Autodesk Inventor part; units mm, degrees
ref_plane "YZ Plane" through (0, 0, 0) normal (1, 0, 0) x (0, 1, 0)
ref_plane "XZ Plane" through (0, 0, 0) normal (0, 1, 0) x (-1, 0, 0)
ref_plane "XY Plane" through (0, 0, 0) normal (0, 0, 1) x (1, 0, 0)
sketch "Sketch1" plane through (0, 0, 0) normal (0, 1, 0) x (-1, 0, 0)
  line L0 (-25.4, -7.9375) -> (25.4, -7.9375)
  line L1 (25.4, -7.9375) -> (25.4, 7.9375)
  line L2 (25.4, 7.9375) -> (-25.4, 7.9375)
  line L3 (-25.4, 7.9375) -> (-25.4, -7.9375)
  line L4 (-25.4, -7.9375) -> (25.4, 7.9375) construction
  line L5 (25.4, -7.9375) -> (-25.4, 7.9375) construction
  point P0 (0, 0)
  dimension "d0" = 50.8
  dimension "d1" = 15.875
extrude "Extrusion1" add sketch "Sketch1" along normal blind 9.525
sketch "Sketch2" plane through (-25.4, 0, -7.9375) normal (-1, 0, 0) x (0, 0, 1)
  line L0 (0, 9.525) -> (15.875, 9.525)
  line L1 (9.5418, 3.175) -> (6.3668, 3.175)
  line L2 (6.3668, 3.175) -> (6.3668, 9.525)
  line L3 (6.3668, 9.525) -> (9.5418, 9.525)
  line L4 (9.5418, 9.525) -> (9.5418, 3.175)
  line L5 (9.5418, 3.175) -> (6.3668, 9.525) construction
  line L6 (6.3668, 3.175) -> (9.5418, 9.525) construction
  point P0 (7.9375, 0)
  point P1 (7.9543, 6.35)
  dimension "d4" = 3.175
  dimension "d5" = 6.35
extrude "Extrusion2" cut sketch "Sketch2" against normal up to next
properties part number "Test1"
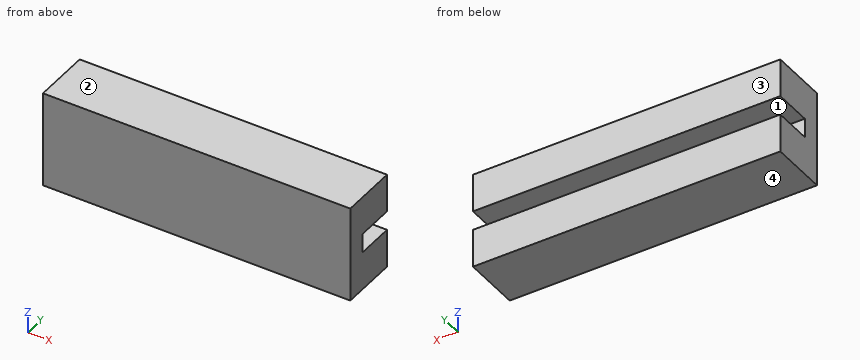
The model under review builds one solid part; all positions refer to its coordinate system, in mm. Face numbers are marked on the shaded views. Round coordinates to 2 decimals unless told otherwise and drop trailing zeros. Order: outer loops, then holes, each group sorted by start corner. A loop starts at its lowest first (then second) coordinate and runs counter-clockwise, first axis right, second up. Notation, with made-up numbers: (86.25, 26.25) -> (127.25, 26.25) arc R24 ccw to (127.25, 62.25) -> close; hole circle Ø9 at (0, -35). An arc over 180 degrees is marked (long way). One line per item, written item: value. Start each with the question number.
Q1. Wall thickness on line 1 (Z direction, x = 16, y = 8.75); line 2 (Y direction, x = -3, z = 1.5) (3 decimals): over which ranges is each line inside the solid? List them lowest first.
Q2. Clearance check with flat-ended pins moving along their axes: pin 1 Ø1.6 at (x, z) = (-9, -0.5) entering from +Y (3 decimals); pin 2 Ø8 at (x, z) = (3.5, -4.5) entering from -Y. State where each tip first meets the part, or that it passes through.
Q3. Take a section at C-C (z = -0.75). Write out the cut boundary in (x, y) (3 decimals).
Q4. Take a section at A-A (y = 8.5). Write out the cut boundary in (x, z), and give its area (3 significant figures).
Q5. Mouldability with a two-part tool opening along Z and no side actions: class the marked faces 1, 2, 3 and 4 as released by +Z, released by -Z, zero draft, split by the parting line, or undercut.
Q6. Take a section at B-B (x = -8). Write out the cut boundary in (y, z) (1 decimal).
Reported:
1. line 1: z = -7.94 to -1.57, 1.6 to 7.94
1. line 2: y = 0 to 3.175
2. pin 1: stops at y = 3.175
2. pin 2: stops at y = 0
3. outline: (-25.4, 0) -> (25.4, 0) -> (25.4, 3.175) -> (-25.4, 3.175) -> close
4. outline: (-25.4, -7.94) -> (25.4, -7.94) -> (25.4, -1.57) -> (-25.4, -1.57) -> close; (-25.4, 1.6) -> (25.4, 1.6) -> (25.4, 7.94) -> (-25.4, 7.94) -> close
4. area: 645 mm2
5. face 1: undercut
5. face 2: released by +Z
5. face 3: zero draft
5. face 4: released by -Z
6. outline: (0, -7.9) -> (9.5, -7.9) -> (9.5, -1.6) -> (3.2, -1.6) -> (3.2, 1.6) -> (9.5, 1.6) -> (9.5, 7.9) -> (0, 7.9) -> close
